Source: CAD feature listing. Evaluate the final solid. Frame: model axes, mm. Face numbers are marked on the shaded views. Coordinates: 2 decimals unless noted, no trailing zeros. Loops run counter-clockwise (first coordinate to the right, second up) from the corner with the lowest first, then second, coordinate; pieces in that order, holes last. Notation, with made-up numbers: M 27,22.5 L 76,22.5 A21 cw 76,57.5 Z; hole C 14,-13 d11. An arc over 180 degrees is marked long. Write each question's results on one line, items separated by ' | '. Start each with the question number.
from build123d import *

# Parameters (mm, degrees)
SKETCH1_R                                  = 17.5
SKETCH1_R_2                                = 15.9125
BOSS_EXTRUDE1_DEPTH                        = 40
SKETCH5_W                                  = 2.75
SKETCH5_H                                  = 17.5
MIRROR1_AT_THE_SECOND_PLANE_COPY_1_SKETC_W = 2.75
MIRROR1_AT_THE_SECOND_PLANE_COPY_1_SKETC_H = 17.5


with BuildPart() as part:
    # Sketch1 → Boss-Extrude1 (new body, symmetric)
    with BuildSketch(Plane.XY):
        Circle(SKETCH1_R)
        Circle(SKETCH1_R_2, mode=Mode.SUBTRACT)
    extrude(amount=BOSS_EXTRUDE1_DEPTH, both=True)

    # Sketch5 → M5 Clearance Hole1 (revolve, cut)
    with BuildSketch(Plane(origin=(0, 0, -20), x_dir=(0, 0, -1), z_dir=(1, 0, 0))):
        with Locations((1.375, 8.75)):
            Rectangle(SKETCH5_W, SKETCH5_H)
    m5_clearance_hole1 = revolve(axis=Axis((0, -6.35, -20), (0, 1, 0)), mode=Mode.SUBTRACT)

    # Mirror1: M5 Clearance Hole1 across plane
    add(m5_clearance_hole1.mirror(Plane.XY), mode=Mode.SUBTRACT)

    # Mirror1 at the second plane: M5 Clearance Hole1 across plane
    add(m5_clearance_hole1.mirror(Plane.ZX), mode=Mode.SUBTRACT)

    # Mirror1 at the second plane copy 1 sketc → Mirror1 at the second plane copy 1 (revolve, cut)
    with BuildSketch(Plane(origin=(0, 0, 20), x_dir=(0, 0, 1), z_dir=(1, 0, 0))):
        with Locations((1.375, 8.75)):
            Rectangle(MIRROR1_AT_THE_SECOND_PLANE_COPY_1_SKETC_W, MIRROR1_AT_THE_SECOND_PLANE_COPY_1_SKETC_H)
    revolve(axis=Axis((0, 6.35, 20), (0, -1, 0)), mode=Mode.SUBTRACT)


solid = part.part
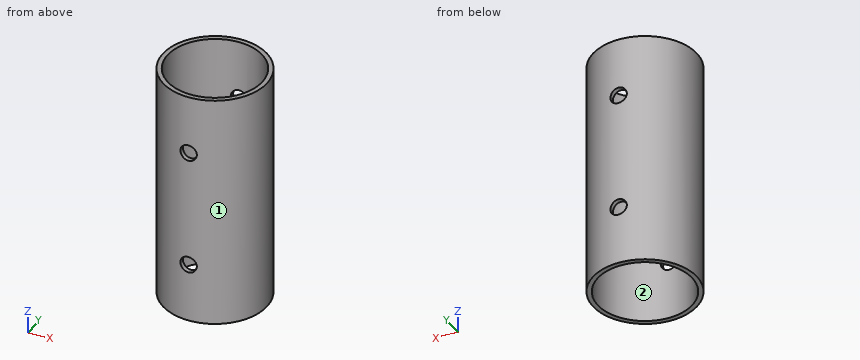
Item 1: Line query: probe 1 along Z at (x, y) = (0, -16.9); probe 2 along Y at (x, z) = (0, -11); probe 3 along Y at (x, z) = (-13, 32). Output: solid intervals per line, ascending.
Item 2: Cut plane B-B (x = -13.5). Output: boundary loops of the cut face in (y, z), then the cut area to 3 significant figures.
Item 3: First-contact query: pin 1 Ø1 at (y, z) = (-10.5, 29) entering from -X; pin 2 Ø9 at (x, z) = (0, -20) entering from +Y; pin 3 Ø2 at (y, z) = (-12, 31.5) entering from -X; pin 4 Ø1.5 at (y, z) = (5, -17) entering from +X. Flat tips, straight axial feed; report the tip coordinate or a pass-through.
Item 4: Cut plane A-A (y = 0). Output: boundary loops of the cut face in (x, z), then the cut area to 3 significant figures.
Item 5: Cut plane C-C (x = 0). Output: boundary loops of the cut face in (y, z), then the cut area to 3 significant figures.
Item 6: Mould query, pull axis Y, two halves, no side actions, for the marked faces 1 and 2. Classes: +Y half, -Y half, draft (parallel to the pull), parting line (faces both ways), or undercut.
Item 7: Cut plane D-D (z = 25.5). Output: boundary loops of the cut face in (x, y) (1 decimal), then the cut area to 3 significant figures.
Response values:
1) probe 1: z = -40 to -22.75, -17.25 to 17.25, 22.75 to 40 | probe 2: y = -17.5 to -15.91, 15.91 to 17.5 | probe 3: y = -11.72 to -9.18, 9.18 to 11.72
2) outline: M -11.14,-40 L -8.42,-40 L -8.42,40 L -11.14,40 Z; M 8.42,-40 L 11.14,-40 L 11.14,40 L 8.42,40 Z | area: 434 mm2
3) pin 1: stops at x = -14.36 | pin 2: stops at y = 17.5 | pin 3: stops at x = -13.61 | pin 4: stops at x = 16.98
4) outline: M -17.5,-40 L -15.91,-40 L -15.91,40 L -17.5,40 Z; M 15.91,-40 L 17.5,-40 L 17.5,40 L 15.91,40 Z | area: 254 mm2
5) outline: M -17.5,-40 L -15.91,-40 L -15.91,-22.75 L -17.5,-22.75 Z; M -17.5,-17.25 L -15.91,-17.25 L -15.91,17.25 L -17.5,17.25 Z; M -17.5,22.75 L -15.91,22.75 L -15.91,40 L -17.5,40 Z; M 15.91,-40 L 17.5,-40 L 17.5,-22.75 L 15.91,-22.75 Z; M 15.91,-17.25 L 17.5,-17.25 L 17.5,17.25 L 15.91,17.25 Z; M 15.91,22.75 L 17.5,22.75 L 17.5,40 L 15.91,40 Z | area: 219 mm2
6) face 1: parting line | face 2: undercut
7) outline: C 0,0 d35; hole C 0,0 d31.8 | area: 167 mm2
